from build123d import *

# Parameters (mm, degrees)
SKETCH1_W           = 40
SKETCH1_H           = 40
BOSS_EXTRUDE1_DEPTH = 3.175
SKETCH3_W           = 15
SKETCH3_H           = 10
SKETCH3_W_2         = 10
CUT_EXTRUDE2_DEPTH  = 10
SKETCH4_R           = 1.6
CUT_EXTRUDE3_DEPTH  = 29.461915343
SKETCH5_W           = 10
SKETCH5_H           = 5
CUT_EXTRUDE4_DEPTH  = 10
SKETCH7_R           = 1.6
CUT_EXTRUDE6_DEPTH  = 10
SKETCH8_W           = 15
SKETCH8_H           = 34.175
BOSS_EXTRUDE2_DEPTH = 3.175
SKETCH9_R           = 1.6
CUT_EXTRUDE7_DEPTH  = 32.535872431
SKETCH10_W          = 5
SKETCH10_H          = 25
CUT_EXTRUDE8_DEPTH  = 10
FILLET1_R           = 1


with BuildPart() as part:
    # Sketch1 → Boss-Extrude1 (new body)
    with BuildSketch(Plane(origin=(0, 0, 0), x_dir=(1, 0, 0), z_dir=(0, 1, 0))):
        Rectangle(SKETCH1_W, SKETCH1_H)
    extrude(amount=BOSS_EXTRUDE1_DEPTH)

    # Sketch3 → Cut-Extrude2 (cut)
    with BuildSketch(Plane(origin=(0, 3.175, 0), x_dir=(1, 0, 0), z_dir=(0, 1, 0))):
        with Locations((-12.5, 15)):
            Rectangle(SKETCH3_W, SKETCH3_H)
        with Locations((15, 15)):
            Rectangle(SKETCH3_W_2, SKETCH3_H)
    extrude(amount=-CUT_EXTRUDE2_DEPTH, mode=Mode.SUBTRACT)

    # Sketch4 → Cut-Extrude3 (cut, through all)
    with BuildSketch(Plane(origin=(0, 3.175, 0), x_dir=(1, 0, 0), z_dir=(0, 1, 0))):
        with Locations(Location((2.5, 17, 0), (0, 0, 270))):
            Circle(SKETCH4_R)
    extrude(amount=-CUT_EXTRUDE3_DEPTH, mode=Mode.SUBTRACT)

    # Sketch5 → Cut-Extrude4 (cut)
    with BuildSketch(Plane(origin=(0, 3.175, 0), x_dir=(1, 0, 0), z_dir=(0, 1, 0))):
        with Locations((-15, 7.5)):
            Rectangle(SKETCH5_W, SKETCH5_H)
        Polygon((-10, -20), (-20, -20), (-20, -10), (-10, -10), (-10, -15), (20, -15), (20, -20), align=None)
    extrude(amount=-CUT_EXTRUDE4_DEPTH, mode=Mode.SUBTRACT)

    # Sketch7 → Cut-Extrude6 (cut)
    with BuildSketch(Plane(origin=(0, 3.175, 0), x_dir=(1, 0, 0), z_dir=(0, 1, 0))):
        with Locations(Location((-17, -2.5, 0), (0, 0, 270))):
            Circle(SKETCH7_R)
    extrude(amount=-CUT_EXTRUDE6_DEPTH, mode=Mode.SUBTRACT)

    # Sketch8 → Boss-Extrude2 (add)
    with BuildSketch(Plane(origin=(0, 3.175, 0), x_dir=(1, 0, 0), z_dir=(0, 1, 0))):
        with Locations((2.5, -7.0875)):
            Rectangle(SKETCH8_W, SKETCH8_H)
    extrude(amount=-BOSS_EXTRUDE2_DEPTH)

    # Sketch9 → Cut-Extrude7 (cut, through all)
    with BuildSketch(Plane(origin=(0, 3.175, 0), x_dir=(1, 0, 0), z_dir=(0, 1, 0))):
        with Locations(Location((2.5, -21.175, 0), (0, 0, 270))):
            Circle(SKETCH9_R)
    extrude(amount=-CUT_EXTRUDE7_DEPTH, mode=Mode.SUBTRACT)

    # Sketch10 → Cut-Extrude8 (cut)
    with BuildSketch(Plane(origin=(0, 3.175, 0), x_dir=(1, 0, 0), z_dir=(0, 1, 0))):
        with Locations((17.5, -2.5)):
            Rectangle(SKETCH10_W, SKETCH10_H)
    extrude(amount=-CUT_EXTRUDE8_DEPTH, mode=Mode.SUBTRACT)

    # Fillet1
    fillet1_edges = [part.edges().sort_by_distance(p)[0] for p in [
        (-5, 1.5875, 24.175),
        (10, 1.5875, 24.175),
        (15, 1.5875, 15),
        (15, 1.5875, -10),
        (-5, 1.5875, -20),
        (10, 1.5875, -20),
        (-10, 1.5875, -10),
        (-20, 1.5875, -5),
        (-20, 1.5875, 10),
        (-10, 1.5875, 15),
    ]]
    fillet(fillet1_edges, radius=FILLET1_R)


solid = part.part
The model under review builds one solid part; all positions refer to its coordinate system, in mm. A direction names the side the tool comes from. Give positions to 0.01 mm unless a question says otherwise; leave off trailing zeros. Loops run counter-clockwise (first coordinate to the right, second up) from the corner with the lowest first, then second, coordinate; pieces in that order, holes last. Notation, with made-up numbers: (54.5, 40.5) -> (83.5, 40.5) arc R15 ccw to (83.5, 46.5) -> close; hole circle Ø8 at (4.5, 68.5). An arc over 180 degrees is marked (long way). Answer as a JSON object with one key per item and string values. Group by question number.
Q1. Take a section at A-A (z = 2.5). Write out the cut boundary in (x, y) (3 decimals).
Q2. Take a section at D-D (y = 0.75). State how many separate pieces and enclosed holes the cut face has, plus the area to 3 significant figures.
Q3. Draft analysis for pull direction X (two halves, no side actions). For faces 6 (the cylindrical face through (14.715, 1.565, 14.699)), 7 (the cylindrical face through (2.57, 1.61, 19.577)), 8 (the flat face through (2, 2, -20)), 9 (the cylindrical face through (2.57, 1.61, -18.6)), state which applies: pulls with the +X half, pulls with the -X half, needs draft (parallel to the pull), parting line crosses it, or undercut.
Q4. Take a section at B-B (x = 2.5). Write out the cut boundary in (y, z) (3 decimals).
Q5. Take a section at C-C (x = -17). Write out the cut boundary in (y, z) (3 decimals), plus the area to 3 significant figures.
Q6. Tool access review of faces 1 (the cylindrical face through (9.7, 1.57, 23.89)), 2 (the flat face through (10, 2, -14)), 3 (the flat face through (-10, 2, -7)), 4 (the flat face through (-15, 2, 10)), 5 (the flat face through (1, 3.175, 2)): name each direction out of +Z, -Z, +X, -X, +Y, -Y from which nothing blocks a thin tool from reaching the whole face with its end or side.
Q7. Wall thickness on line 1 along Z through (x, y) = (3.5, 2.25) (3 decimals); line 2 along X through (y, z) = (2.45, 22); line 3 along Z through (x, y) = (-12, 1.6): over which ranges is each line inside the solid? List them lowest first.
Q8. Insertion check: pin 1 (1 mm diameter, centred on y = 2.5, z = -7, fed in from -X); pin 2 (1.6 mm diameter, centred on x = 12, y = 1.5, fed in from -Z); pin 3 (1 mm diameter, centred on x = -7, y = 1.5, fed in from +Z); pin 4 (3 mm diameter, centred on x = -17, z = 2.5, fed in from -Y). Each pin has a flat end and moves straight along its axis. Give the tip position at first contact, or say it passes through.
Answer below:
{
 "1": {"outline": "(-20, 0) -> (-18.6, 0) -> (-18.6, 3.175) -> (-20, 3.175) -> close; (-15.4, 0) -> (15, 0) -> (15, 3.175) -> (-15.4, 3.175) -> close"},
 "2": {"separate pieces": "1", "enclosed holes": "3", "area": "1,040 mm2"},
 "3": {"face 6": "pulls with the +X half", "face 7": "undercut", "face 8": "needs draft", "face 9": "undercut"},
 "4": {"outline": "(0, -20) -> (3.175, -20) -> (3.175, -18.6) -> (0, -18.6) -> close; (0, -15.4) -> (3.175, -15.4) -> (3.175, 19.575) -> (0, 19.575) -> close; (0, 22.775) -> (3.175, 22.775) -> (3.175, 24.175) -> (0, 24.175) -> close"},
 "5": {"outline": "(0, -5) -> (3.175, -5) -> (3.175, 0.9) -> (0, 0.9) -> close; (0, 4.1) -> (3.175, 4.1) -> (3.175, 10) -> (0, 10) -> close", "area": "37.5 mm2"},
 "6": {"face 1": "+Z, +X, +Y, -Y", "face 2": "-Z, +X, +Y, -Y", "face 3": "-Z, -X, +Y, -Y", "face 4": "+Z, -X, +Y, -Y", "face 5": "+Z, -Z, +X, -X, +Y"},
 "7": {"line 1": "z = -20 to -18.249, -15.751 to 19.926, 22.424 to 24.175", "line 2": "x = -5 to 1.13, 3.87 to 10", "line 3": "z = -5 to 10"},
 "8": {"pin 1": "stops at x = -10", "pin 2": "stops at z = -10", "pin 3": "stops at z = 15", "pin 4": "passes through"}
}
